from build123d import *

# Parameters (mm, degrees)
F0_W     = 55.978216
F0_H     = 30.363508
F0_R     = 5.489689
F0_R_2   = 5.372442
F1_DEPTH = 5
F3_DEPTH = 6.1
F4_R     = 6.25311
F5_DEPTH = 25


with BuildPart() as f1:
    # F0 (on Front) → F1 (new body)
    with BuildSketch(Plane.XZ):
        with Locations((27.989108, 15.181754)):
            Rectangle(F0_W, F0_H)
        with Locations((13.994554, 15.181754)):
            Circle(F0_R, mode=Mode.SUBTRACT)
        with Locations((41.983662, 15.181754)):
            Circle(F0_R_2, mode=Mode.SUBTRACT)
    extrude(amount=F1_DEPTH)

    # F2 (on face) → F3 (join)
    with BuildSketch(Plane.YZ.offset(55.978216)):
        with BuildLine():
            Line((10.672215, 30.363508), (0, 30.363508))
            Line((0, 30.363508), (-5, 30.363508))
            Line((-5, 30.363508), (-5, 0))
            Line((-5, 0), (0, 0))
            Line((0, 0), (10.672215, 0))
            ThreePointArc((10.672215, 0), (25.853969, 15.181754), (10.672215, 30.363508))
        make_face()
    extrude(amount=F3_DEPTH)

    # F4 (on face) → F5 (cut)
    with BuildSketch(Plane(origin=(55.978216, 0, 0), x_dir=(0, -1, 0), z_dir=(-1, 0, 0))):
        with Locations((-10.672215, 15.181754)):
            Circle(F4_R)
    extrude(amount=-F5_DEPTH, mode=Mode.SUBTRACT)


solid = f1.part
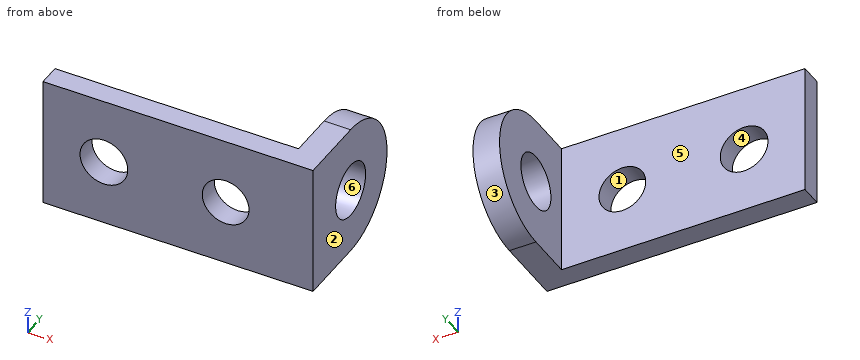
Check sheet for the modelled part. Datum: model origin and axes. Units: mm. Face numbers are marked on the shaded views. A direction names the side the tool comes from. Round coordinates to 2 decimals unless told otherwise and drop trailing zeros. Order: outer loops, then holes, each group sorted by start corner. A loop starts at its lowest first (then second) coordinate and runs counter-clockwise, first axis right, second up.
(1) Cross-section at A-A, the plane x = 11.5. Enter the section's corners in (y, z).
(2) Access from +Z, -Z, +X, -X, +Y, -Y to the whole of each face (thin tool, end or side, straight path). Record for the marked faces 5 and 6.
(3) Draft check along X on the marked faces 1, 2, 3 and 4. Enter one of: pulls with the +X half, pulls with the -X half, needs draft (parallel to the pull), parting line crosses it, or undercut.
(4) Cross-section at D-D, the plane z = 24. Enter the section's corners in (x, y).
(5) Go/stop test with flat-tipped pins: P1, Ø1, axis at y = -1.5, z = 25.5, coming from the -X side; P2, Ø12, axis at y = 20.5, z = 22, coming from the -X side; P3, Ø15, axis at x = 42, z = 13.5, coming from the +Y side. Record where each tip stops, or that it passes through.
(6) Cross-section at B-B, the plane z = 18. Enter the section's corners in (x, y), and give its area (3 significant figures).
(7) Scan lines: probe 1 along Y at (x, z) = (53, 28); probe 2 along X at (y, z) = (0.5, 23.5). Record each from-to range of solid material in increasing order.
(8) Cross-section at C-C, the plane y = 6. Enter the section's corners in (x, z).
Check sheet entries:
1. outline: (-5, 0) - (0, 0) - (0, 10.29) - (-5, 10.29) - close; (-5, 20.07) - (0, 20.07) - (0, 30.36) - (-5, 30.36) - close
2. face 5: +Z, -Z, -X, +Y
2. face 6: +X, -X
3. face 1: undercut
3. face 2: pulls with the +X half
3. face 3: needs draft
3. face 4: undercut
4. outline: (0, -5) - (62.08, -5) - (62.08, 23.03) - (55.98, 23.03) - (55.98, 0) - (0, 0) - close
5. P1: stops at x = 0
5. P2: stops at x = 55.98
5. P3: stops at y = 0
6. outline: (0, -5) - (9.28, -5) - (9.28, 0) - (0, 0) - close; (18.71, -5) - (37.41, -5) - (37.41, 0) - (18.71, 0) - close; (46.56, -5) - (62.08, -5) - (62.08, 5.09) - (55.98, 5.09) - (55.98, 0) - (46.56, 0) - close; (55.98, 16.25) - (62.08, 16.25) - (62.08, 25.59) - (55.98, 25.59) - close
6. area: 306 mm2
7. probe 1: y = -5 to 0
7. probe 2: x = 55.98 to 62.08
8. outline: (55.98, 0) - (62.08, 0) - (62.08, 11.03) - (55.98, 11.03) - close; (55.98, 19.34) - (62.08, 19.34) - (62.08, 30.36) - (55.98, 30.36) - close
